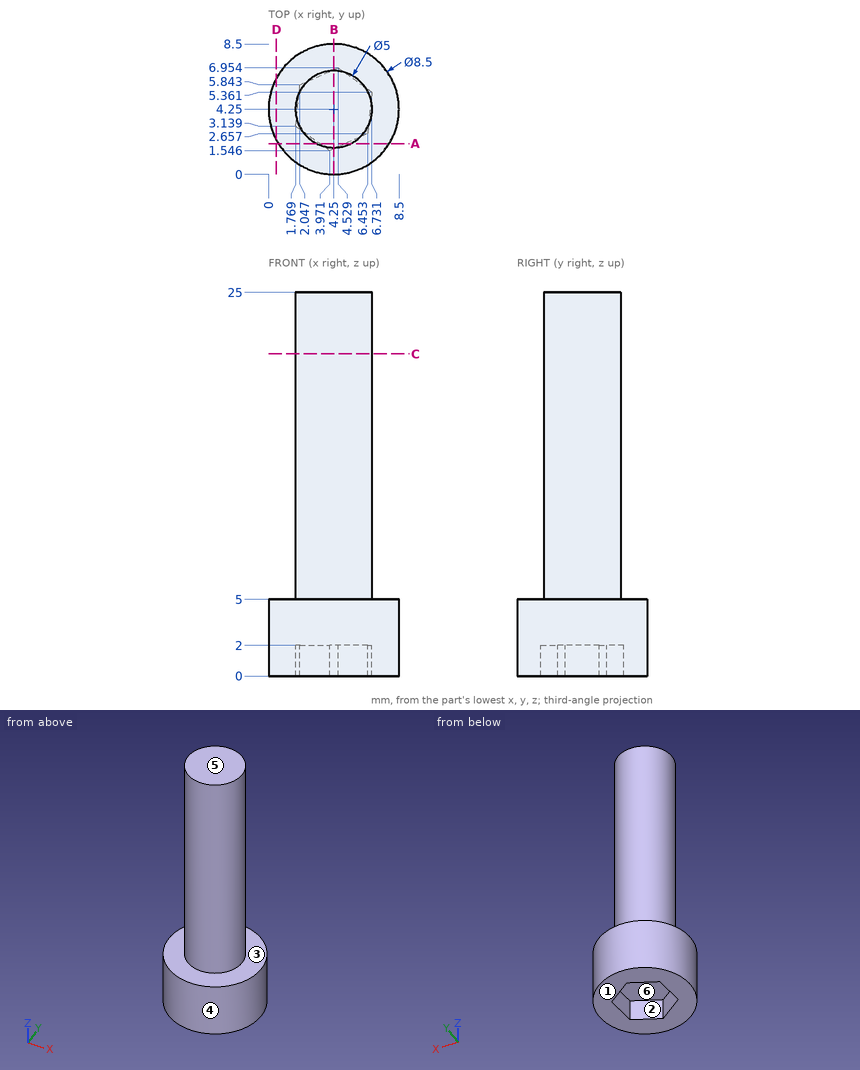
Design review of the part shown in the three views and the two pictorial views. Dimensions are in mm from the part's minimum x, y and z. A direction names the side the tool comes from. Round coordinates to 2 decimals unless told otherwise and drop trailing zeros. Write each loop counter-clockwise with the first axis right and the second up, starting at its lowest first coordinate (ties: lowest second). Pieces come first, ordered by that corner, then holes.
Item 1: The part is to be moulded in two halves that separate along X. For the marked faces 4, 5 and 6, say which applies: +X half, -X half, draft (parallel to the pull), parting line (faces both ways), or undercut.
Item 2: We need section D-D on x = 0.5. Write out the cut boundary in (y, z).
Item 3: Clearance check with flat-ended pins moving along their axes: pin 1 Ø2 at (y, z) = (3.5, 21.5) entering from -X; pin 2 Ø1.5 at (x, z) = (6, 14) entering from -Y; pin 3 Ø1.5 at (x, z) = (6.5, 20) entering from -Y. State where each tip first meets the part, or that it passes through.
Item 4: We need section C-C on z = 21. Write out the cut boundary in (x, y).
Item 5: We need section B-B on x = 4.25. Write out the cut boundary in (y, z).
Item 6: For probe 1 along Z at (x, y) = (5.5, 7.75); probe 2 along Z at (x, y) = (4.5, 5.5); probe 3 along X at (y, z) = (4, 19), list the stretches that pass through material, from the lowest coordinate up.
Item 7: We need section A-A on y = 2. Write out the cut boundary in (x, z) (1 decimal).
Item 8: For the marked faces 1, 2 and 3, list the 3-axis set-ups (+Z, -Z, +X, -X, +Y, -Y) from which the entire face can be reached by the end or side of a thin tool; tool diameter is ignored.
Returned:
1. face 4: parting line
1. face 5: draft
1. face 6: undercut
2. outline: (2.25, 0) - (6.25, 0) - (6.25, 5) - (2.25, 5) - close
3. pin 1: stops at x = 1.75
3. pin 2: stops at y = 1.96
3. pin 3: stops at y = 2.25
4. outline: circle Ø5 at (4.25, 4.25)
5. outline: (0, 0) - (1.67, 0) - (1.67, 2) - (6.83, 2) - (6.83, 0) - (8.5, 0) - (8.5, 5) - (6.75, 5) - (6.75, 25) - (1.75, 25) - (1.75, 5) - (0, 5) - close
6. probe 1: z = 0 to 5
6. probe 2: z = 2 to 25
6. probe 3: x = 1.76 to 6.74
7. outline: (0.6, 0) - (3.3, 0) - (3.3, 2) - (5, 2) - (5, 0) - (7.9, 0) - (7.9, 5) - (5.3, 5) - (5.3, 25) - (3.2, 25) - (3.2, 5) - (0.6, 5) - close
8. face 1: -Z, +X, -X, +Y, -Y
8. face 2: -Z
8. face 3: +Z
